CAD build for the part. Positions are in the model's coordinates, mm. Face numbers are marked on the shaded views. A direction names the side the tool comes from. Give positions to 0.01 mm unless a question says otherwise; leave off trailing zeros. Loops run counter-clockwise (first coordinate to the right, second up) from the corner with the lowest first, then second, coordinate; pieces in that order, holes last. Notation, with made-up numbers: M -29.75,87 L 11.25,87 A8 ccw 11.25,92 Z; hole C 61,-16 d7. An arc over 180 degrees is marked long. Answer as CSV lines item,"result".
```python
from build123d import *

# Parameters (mm, degrees)
F0_R         = 4.15
F1_DEPTH     = 15
F2_W         = 14
F2_H         = 15
F3_DEPTH     = 4
F4_R         = 3.85
F5_DEPTH     = 3
F6_T1_DEPTH  = 40.5779464854
F4_R_2       = 1.6
F7_DEPTH     = 7
F8_DEPTH     = 0.6
F10_DEPTH    = 25
F11_T1_DEPTH = 30.4300979278
F11_T3_DEPTH = 10.4650489639
F11_T5_DEPTH = 10.4650489639


# Not quite as in the source:
# - a fillet or chamfer that OpenCascade refuses, or shapes differently, is made with other operations: its cross-section is extruded or revolved along the edge and cut away or added


with BuildPart() as f1:
    # F0 (on Top) → F1 (new body)
    with BuildSketch(Plane.XY):
        with BuildLine():
            Line((7, 7), (-27.5, 7))
            ThreePointArc((-27.5, 7), (-34.5, 0), (-27.5, -7))
            Line((-27.5, -7), (7, -7))
            Line((7, -7), (7, 7))
        make_face()
        with Locations((-27.5, 0)):
            Circle(F0_R, mode=Mode.SUBTRACT)
        Circle(F0_R, mode=Mode.SUBTRACT)
    extrude(amount=F1_DEPTH)

    # F2 (on face) → F3 (join)
    with BuildSketch(Plane.XZ.offset(7)):
        with Locations((0, 7.5)):
            Rectangle(F2_W, F2_H)
    extrude(amount=F3_DEPTH)

    # F4 (on face) → F5 (join)
    with BuildSketch(Plane.XZ.offset(11)):
        with BuildLine():
            ThreePointArc((0, 2.75), (3.3587572106, 4.1412427894), (4.75, 7.5))
            ThreePointArc((4.75, 7.5), (3.3587572106, 10.8587572106), (0, 12.25))
            ThreePointArc((0, 12.25), (-4.75, 7.5), (0, 2.75))
        make_face()
        with Locations((0, 7.5)):
            Circle(F4_R, mode=Mode.SUBTRACT)
        with BuildLine():
            ThreePointArc((0, 12.25), (3.3587572106, 10.8587572106), (4.75, 7.5))
            ThreePointArc((4.75, 7.5), (3.3587572106, 4.1412427894), (0, 2.75))
            Line((0, 2.75), (18, 2.75))
            Line((18, 2.75), (18, 12.25))
            Line((18, 12.25), (0, 12.25))
        make_face()
        with BuildLine():
            ThreePointArc((0, 2.75), (-4.75, 7.5), (0, 12.25))
            Line((0, 12.25), (-18, 12.25))
            Line((-18, 12.25), (-18, 2.75))
            Line((-18, 2.75), (0, 2.75))
        make_face()
    extrude(amount=-F5_DEPTH)

    # F6: chamfer of 3 x 6 on 2 edges, made by hand

    # F6_s2 → F6_t1 (cut)
    with BuildSketch(Plane.XY.offset(-12.7889732427)):
        Polygon((-12, -8), (-18, -11), (-18, -8), align=None)
        Polygon((12, -8), (18, -11), (18, -8), align=None)
    extrude(amount=F6_T1_DEPTH, mode=Mode.SUBTRACT)

    # F4 (on face) → F7 (join)
    with BuildSketch(Plane.XZ.offset(11)):
        with Locations((0, 7.5)):
            Circle(F4_R)
        with Locations((0, 7.5)):
            Circle(F4_R_2, mode=Mode.SUBTRACT)
    extrude(amount=F7_DEPTH)

    # F4 (on face) → F8 (join)
    with BuildSketch(Plane.XZ.offset(11)):
        with BuildLine():
            ThreePointArc((0, 2.75), (3.3587572106, 4.1412427894), (4.75, 7.5))
            ThreePointArc((4.75, 7.5), (3.3587572106, 10.8587572106), (0, 12.25))
            ThreePointArc((0, 12.25), (-4.75, 7.5), (0, 2.75))
        make_face()
        with Locations((0, 7.5)):
            Circle(F4_R, mode=Mode.SUBTRACT)
    extrude(amount=F8_DEPTH)

    # F9 (on face) → F10 (intersect, symmetric)
    with BuildSketch(Plane.XZ.offset(7)):
        with BuildLine():
            Line((-27.5, 6.2586253838), (-27.5, 0))
            Line((-27.5, 0), (-7, 0))
            Line((-7, 0), (-7, 15))
            Line((-7, 15), (-9, 15))
            add(Edge.make_bspline(
                [(-27.5, 6.2586253838), (-22.0570868036, 9.2486118384), (-19.3657420182, 15), (-9, 15)],
                knots=[7.0475438496, 7.0475438496, 7.0475438496, 7.0475438496, 27.5771644663, 27.5771644663, 27.5771644663, 27.5771644663], degree=3))
        make_face()
        with BuildLine():
            Line((-34.5, 4.5), (-34.5, 0))
            Line((-34.5, 0), (-27.5, 0))
            Line((-27.5, 0), (-27.5, 6.2586253838))
            add(Edge.make_bspline(
                [(-34.5, 4.5), (-31.5612189253, 4.5312000669), (-29.3684792153, 5.2322030722), (-27.5, 6.2586253838)],
                knots=[0, 0, 0, 0, 7.0475438496, 7.0475438496, 7.0475438496, 7.0475438496], degree=3))
        make_face()
        Polygon((-7, 15), (-7, 0), (0, 0), (17, 0), (17, 15), align=None)
    extrude(amount=F10_DEPTH, both=True, mode=Mode.INTERSECT)

    # F11: chamfer of 3 on 6 edges, made by hand

    # F11_s2 → F11_t1 (cut)
    with BuildSketch(Plane.XY.offset(-7.7150489639)):
        Polygon((4, 7), (7, 4), (7, 7), align=None)
    extrude(amount=F11_T1_DEPTH, mode=Mode.SUBTRACT)

    # F11_s4 → F11_t3 (cut)
    with BuildSketch(Plane.XY.offset(12.25)):
        Polygon((-4, -11), (-7, -8), (-7, -11), align=None)
        Polygon((7, -8), (4, -11), (7, -11), align=None)
    extrude(amount=F11_T3_DEPTH, mode=Mode.SUBTRACT)

    # F11_s6 → F11_t5 (cut)
    with BuildSketch(Plane.XY.offset(-7.7150489639)):
        Polygon((-4, -11), (-7, -8), (-7, -11), align=None)
        Polygon((7, -8), (4, -11), (7, -11), align=None)
    extrude(amount=F11_T5_DEPTH, mode=Mode.SUBTRACT)


solid = f1.part
```
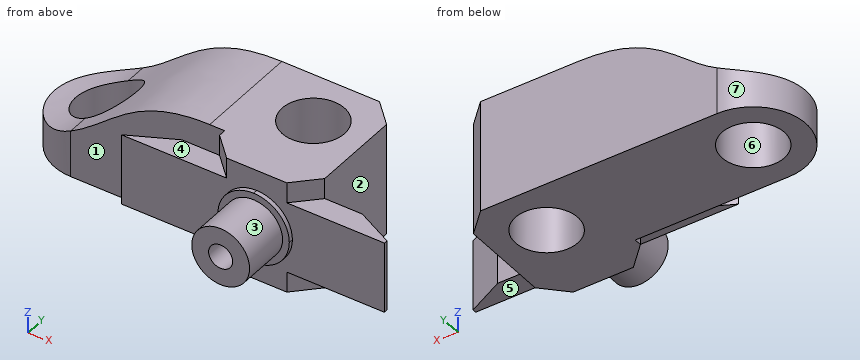
Q1. Cut at C-C (y = -13.5). Write the cut outline in (x, z).
Solution:
outline,"C 0,7.5 d7.7; hole C 0,7.5 d3.2"
Q2. Wall check: line 1 (Y direction, x = -27.5, z = 4.5); line 2 (X direction, y = -3.5, z = 2.75); line 3 (Z direction, x = 0, y = -14). Give the ranges that are in metal, low to high. Write a range as [from, to].
Solution:
line 1,"y = [-7, -4.15], [4.15, 7]"
line 2,"x = [-33.56, -29.73], [-25.27, -2.23], [2.23, 7]"
line 3,"z = [3.65, 5.9], [9.1, 11.35]"
Q3. Cut at A-A (x = 2.5). Write the cut outline in (y, z), and give its area (3 significant figures).
Solution:
outline,"M -18,4.57 L -11.6,4.57 L -11.6,3.46 L -11,3.46 L -11,0 L -3.31,0 L -3.31,15 L -11,15 L -11,11.54 L -11.6,11.54 L -11.6,10.43 L -18,10.43 Z; M 3.31,0 L 7,0 L 7,15 L 3.31,15 Z"
area,"213 mm²"
Q4. Which spindle directions (+Z, -Z, +X, -X, +Y, -Y) get a long thin tool onto all of the face, cutting with end or side? Do the marked faces 1, 2, 3 and 4. Say none if no direction does.
Solution:
face 1,"+Z, -Z, -X"
face 2,"+Z, -Z, +X, +Y"
face 3,"-Y"
face 4,"+Z, -X, -Y"
Q5. Cut at D-D (x = 12.5). Write the cut outline in (y, z), and give its area (3 significant figures).
Solution:
outline,"M -11,2.75 L -8.25,2.75 L -8.25,12.25 L -11,12.25 Z"
area,"26.1 mm²"
Q6. Pin check, flat tips, straight feed: P1, Ø1.5, axis at x = -11, y = -10, coming from the +Z side; P2, Ø6, axis at y = 0.5, z = 5.5, coming from the +X side; P3, Ø1, axis at y = 2, z = 3, coming from the -X side; P4, Ø7.5, axis at x = -27.5, y = 0, coming from the +Z side. Stop position of each tip, or through.
Solution:
P1,"stops at z = 12.25"
P2,"stops at x = 7"
P3,"stops at x = -34.34"
P4,"passes through"
Q7. Mould opens along Y. For the marked faces 5, 6 and 7 say: released by +Y, released by -Y, zero draft, split by the parting line, or undercut.
Solution:
face 5,"zero draft"
face 6,"undercut"
face 7,"split by the parting line"
Q8. Cut at B-B (y = -10). Write the cut outline in (x, z), and give its area (3 significant figures).
Solution:
outline,"M -16,2.75 L -5,2.75 L -5,0 L 5,0 L 5,2.75 L 16,2.75 L 16,12.25 L 5,12.25 L 5,15 L -5,15 L -5,12.25 L -16,12.25 Z"
area,"359 mm²"
